Geometry check sheet. Reference: the model listing, model coordinates, mm. Face numbers are marked on the shaded views. A direction names the side the tool comes from. Coordinates: 2 decimals unless noted, no trailing zeros. Write each loop counter-clockwise with the first axis right and the second up, starting at its lowest first coordinate (ties: lowest second). Pieces come first, ordered by that corner, then holes. Notation, with made-up numbers: (69, 88) - (112, 88) arc R17 cw to (112, 101) - close; hole circle Ø11 at (9, 56). An arc over 180 degrees is marked (long way). Answer as a JSON object with one key per item and string values. Group by question number.
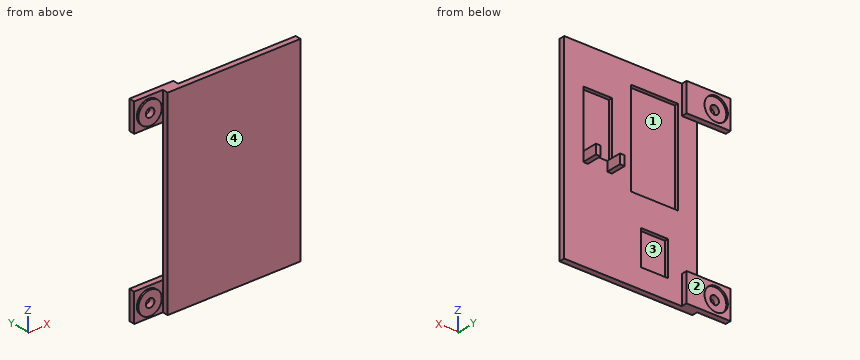
Autodesk Inventor part; units mm, degrees
ref_plane "YZ Plane" through (0, 0, 0) normal (1, 0, 0) x (0, 1, 0)
ref_plane "XZ Plane" through (0, 0, 0) normal (0, 1, 0) x (-1, 0, 0)
ref_plane "XY Plane" through (0, 0, 0) normal (0, 0, 1) x (1, 0, 0)
sketch "Sketch1" plane through (0, 0, 0) normal (0, 1, 0) x (-1, 0, 0)
  line L0 (7.25, 29.75) -> (-17.25, 29.75)
  line L1 (-17.25, 29.75) -> (-17.25, -19.75)
  line L2 (-17.25, -19.75) -> (7.25, -19.75)
  line L3 (7.25, -19.75) -> (7.25, 29.75)
  line L4 (7.25, 29.75) -> (-17.25, -19.75) construction
  line L5 (-17.25, 29.75) -> (7.25, -19.75) construction
  line L6 (-27.25, 20) -> (-42.25, 20)
  line L7 (-42.25, 20) -> (-42.25, -10)
  line L8 (-42.25, -10) -> (-27.25, -10)
  line L9 (-27.25, -10) -> (-27.25, 20)
  line L10 (-27.25, 20) -> (-42.25, -10) construction
  line L11 (-42.25, 20) -> (-27.25, -10) construction
  line L12 (2.1, -34.75) -> (-12.1, -34.75)
  line L13 (-12.1, -34.75) -> (-12.1, -52.95)
  line L14 (-12.1, -52.95) -> (2.1, -52.95)
  line L15 (2.1, -52.95) -> (2.1, -34.75)
  line L16 (2.1, -34.75) -> (-12.1, -52.95) construction
  line L17 (-12.1, -34.75) -> (2.1, -52.95) construction
  line L18 (17.25, 39.75) -> (17.25, -51.55)
  line L19 (17.25, 24.75) -> (17.25, 39.75)
  line L20 (17.25, -36.55) -> (17.25, -51.55)
  line L21 (17.25, 39.75) -> (-52.25, 39.75)
  line L22 (-52.25, 39.75) -> (-52.25, -63.35)
  line L23 (-52.25, -63.35) -> (17.25, -63.35)
  line L24 (17.25, -63.35) -> (17.25, 39.75)
  point P0 (-34.75, 5)
  point P1 (-5, -43.85)
  point P2 (17.25, 0)
  dimension "d0" = 24.5
  dimension "d1" = 49.5
  dimension "d2" = 15
  dimension "d3" = 30
  dimension "d4" = 10
  dimension "d7" = 14.2
  dimension "d8" = 18.2
  dimension "d9" = 15
  dimension "d17" = 10
  dimension "d19" = 103.1
  dimension "d21" = 10
  dimension "d22" = 10
extrude "Extrusion1" add sketch "Sketch1" along normal blind 3 contours L3 L2 L1 L0 | L9 L8 L7 L6 | L15 L14 L13 L12 | L18 L24 L23 L22 L21
sketch "Sketch2" plane through (0, 3, 0) normal (0, 1, 0) x (1, 0, 0)
  line L0 (-7.2398, -29.7311) -> (17.2602, -29.7311)
  line L1 (17.2602, -29.7311) -> (17.2602, 19.7689)
  line L2 (17.2602, 19.7689) -> (-7.2398, 19.7689)
  line L3 (-7.2398, 19.7689) -> (-7.2398, -29.7311)
  line L4 (-7.2398, -29.7311) -> (17.2602, 19.7689) construction
  line L5 (17.2602, -29.7311) -> (-7.2398, 19.7689) construction
  line L6 (27.2602, -19.9811) -> (42.2602, -19.9811)
  line L7 (42.2602, -19.9811) -> (42.2602, 10.0189)
  line L8 (42.2602, 10.0189) -> (27.2602, 10.0189)
  line L9 (27.2602, 10.0189) -> (27.2602, -19.9811)
  line L10 (27.2602, -19.9811) -> (42.2602, 10.0189) construction
  line L11 (42.2602, -19.9811) -> (27.2602, 10.0189) construction
  line L12 (-2.0898, 34.7689) -> (12.1102, 34.7689)
  line L13 (12.1102, 34.7689) -> (12.1102, 52.9689)
  line L14 (12.1102, 52.9689) -> (-2.0898, 52.9689)
  line L15 (-2.0898, 52.9689) -> (-2.0898, 34.7689)
  line L16 (-2.0898, 34.7689) -> (12.1102, 52.9689) construction
  line L17 (12.1102, 34.7689) -> (-2.0898, 52.9689) construction
  line L18 (-17.2398, -39.7311) -> (-17.2398, 51.5689)
  line L19 (-17.2398, -39.7311) -> (-32.2398, -39.7311)
  line L20 (-32.2398, -39.7311) -> (-32.2398, -24.7311)
  line L21 (-32.2398, -24.7311) -> (-17.2398, -24.7311)
  line L22 (-17.2398, -24.7311) -> (-17.2398, -39.7311)
  line L23 (-17.2398, 51.5689) -> (-32.2398, 51.5689)
  line L24 (-32.2398, 51.5689) -> (-32.2398, 36.5689)
  line L25 (-32.2398, 36.5689) -> (-17.2398, 36.5689)
  line L26 (-17.2398, 36.5689) -> (-17.2398, 51.5689)
  line L27 (-17.2398, -39.7311) -> (52.2602, -39.7311)
  line L28 (52.2602, -39.7311) -> (52.2602, 63.3689)
  line L29 (52.2602, 63.3689) -> (-17.2398, 63.3689)
  line L30 (-17.2398, 63.3689) -> (-17.2398, -39.7311)
  point P0 (0, 0)
  point P1 (34.7602, -4.9811)
  point P2 (5.0102, 43.8689)
  point P3 (-17.2398, 0.0189)
  dimension "d25" = 24.5
  dimension "d26" = 49.5
  dimension "d27" = 15
  dimension "d28" = 30
  dimension "d29" = 10
  dimension "d30" = 14.2
  dimension "d31" = 18.2
  dimension "d32" = 15
  dimension "d33" = 15
  dimension "d34" = 15
  dimension "d35" = 15
  dimension "d36" = 15
  dimension "d37" = 10
  dimension "d38" = 11.8
  dimension "d39" = 103.1
  dimension "d40" = 10
  dimension "d41" = 10
extrude "Extrusion2" cut sketch "Sketch2" against normal blind 2 contours L3 L2 L1 L0 | L9 L8 L7 L6 | L15 L14 L13 L12
sketch "Sketch3" plane through (0, 3, 0) normal (0, 1, 0) x (1, 0, 0)
  point P0 (0, 0)
sketch "Sketch4" plane through (0, 3, 0) normal (0, 1, 0) x (1, 0, 0)
  line L0 (29.7102, 15.7954) -> (39.8102, 15.7954)
  line L1 (39.8102, 15.7954) -> (39.8102, 4.2425)
  line L2 (39.8102, 4.2425) -> (29.7102, 4.2425)
  line L3 (29.7102, 4.2425) -> (29.7102, 15.7954)
  line L4 (27.2602, 10.0189) -> (42.2602, 10.0189)
  line L5 (29.7102, 15.7954) -> (39.8102, 4.2425) construction
  line L6 (39.8102, 15.7954) -> (29.7102, 4.2425) construction
  line L7 (27.2602, 10.0189) -> (29.7102, 10.0189)
  line L8 (29.7102, 10.0189) -> (29.7102, 15.0189)
  line L9 (29.7102, 15.0189) -> (27.2602, 15.0189)
  line L10 (27.2602, 15.0189) -> (27.2602, 10.0189)
  line L11 (42.2602, 10.0189) -> (39.8102, 10.0189)
  line L12 (39.8102, 10.0189) -> (39.8102, 15.0189)
  line L13 (39.8102, 15.0189) -> (42.2602, 15.0189)
  line L14 (42.2602, 15.0189) -> (42.2602, 10.0189)
  point P0 (0, 0)
  point P1 (34.7602, 10.0189)
  point P2 (39.8102, 10.0189)
  point P3 (29.7102, 10.0189)
  dimension "d44" = 10.1
  dimension "d45" = 5
  dimension "d46" = 5
extrude "Extrusion3" add sketch "Sketch4" along normal blind 8 contours L3 L4 L10 L9 | L13 L14 L4 L1
sketch "Sketch7" plane through (0, 3, 0) normal (0, 1, 0) x (1, 0, 0)
  line L0 (-17.25, -39.75) -> (-32.25, -39.75)
  line L1 (-32.25, -39.75) -> (-32.25, -24.75)
  line L2 (-32.25, -24.75) -> (-17.25, -24.75)
  line L3 (-17.25, -24.75) -> (-17.25, -39.75)
  line L4 (52.25, 63.35) -> (-17.25, 63.35)
  line L5 (-17.25, 63.35) -> (-32.25, 63.35)
  line L6 (-32.25, 63.35) -> (-32.25, 48.35)
  line L7 (-32.25, 48.35) -> (-17.25, 48.35)
  line L8 (-17.25, 48.35) -> (-17.25, 63.35)
  line L9 (-17.25, -39.75) -> (-9.25, -39.75)
  line L10 (-9.25, -39.75) -> (-9.25, -24.75)
  line L11 (-9.25, -24.75) -> (-17.25, -24.75)
  line L12 (-17.25, -24.75) -> (-17.25, -39.75)
  line L13 (-17.25, 48.35) -> (-9.25, 48.35)
  line L14 (-9.25, 48.35) -> (-9.25, 63.35)
  line L15 (-9.25, 63.35) -> (-17.25, 63.35)
  line L16 (-17.25, 63.35) -> (-17.25, 48.35)
  point P0 (0, 0)
  dimension "d52" = 15
  dimension "d53" = 15
  dimension "d54" = 15
  dimension "d55" = 15
  dimension "d56" = 8
extrude "Extrusion5" add sketch "Sketch7" along normal blind 3
sketch "Sketch8" plane through (0, 6, 0) normal (0, 1, 0) x (1, 0, 0)
  line L0 (-32.25, -24.75) -> (-32.25, -39.75)
  line L1 (-9.25, -24.75) -> (-32.25, -24.75)
  line L2 (-17.25, 63.35) -> (-17.25, -39.75)
  line L3 (-17.25, -24.75) -> (-32.25, -24.75)
  circle A0 centre (-24.75, -32.25) radius 2.25
  circle A1 centre (-24.75, 55.85) radius 2.25
  point P0 (0, 0)
  dimension "d59" = 4.5
  dimension "d60" = 4.5
extrude "Extrusion6" cut sketch "Sketch8" against normal blind 3
sketch "Sketch9" plane through (0, 6, 0) normal (0, 1, 0) x (1, 0, 0)
  circle A0 centre (-24.75, -32.25) radius 2.25
  circle A1 centre (-24.75, -32.25) radius 6.1
  circle A2 centre (-24.75, 55.85) radius 2.25
  circle A3 centre (-24.75, 55.85) radius 6.1
  point P0 (0, 0)
  dimension "d63" = 12.2
  dimension "d64" = 12.2
extrude "Extrusion7" cut sketch "Sketch9" against normal blind 1 contours A0 | A1 | A3
sketch "Sketch10" plane through (0, 3, 0) normal (0, -1, 0) x (1, 0, 0)
  circle A0 centre (-24.75, 32.25) radius 2.25
  circle A1 centre (-24.75, 32.25) radius 6.1
  circle A2 centre (-24.75, -55.85) radius 2.25
  circle A3 centre (-24.75, -55.85) radius 6.1
  point P0 (0, 0)
  dimension "d67" = 12.2
  dimension "d68" = 12.2
extrude "Extrusion8" add sketch "Sketch10" along normal blind 1
properties part number "chrager_adapter"
(1) Material ranges on L1, parallel to Z at x = -24.75, y = 5.3; L2, parallel to Z at x = -24.75, y = 3.55; L3, parallel to Z at x = 29, y = 2, recorded low to high. Write a range as [from, to].
(2) Gauge pin test, flat ends, axial feed: pin 1 (2 mm diameter, centred on y = 2, z = -1, fed in from -X); pin 2 (7.5 mm diameter, centred on x = 37, z = 5.5, fed in from +Y); pin 3 (3.5 mm diameter, centred on y = 5, z = -55.5, fed in from +X); pin 4 (6 mm diameter, centred on y = 7.5, z = -29.5, fed in from -X) (3 decimals). Record the tip position at first contact, or that the pin passes through.
(3) Set-up check for the marked faces 1 and 2: record each of +Z, -Z, +X, -X, +Y, -Y from which the full face is reachable in a straight line by a thin tool's end or side.
(4) Section check A-A (x = -24.75). Count the separate pieces of the cut face and the enclosed holes in it, and give its area (3 significant figures).
(5) Section check B-B (z = -55.85). Record the cut outline in (x, y), and give its area (3 significant figures).
(6) Section check C-C (y = 9.25). Record the cut outline in (x, z).
(7) Section check D-D (z = -38.5). Record the cut outline in (x, y), and give its area (3 significant figures).
(8) Draft check along Z on the marked faces 3 and 4. Enter one of: +Z half, -Z half, draft (parallel to the pull), parting line (faces both ways), or undercut.
Conclusion:
{
 "1": {"L1": "z = [-63.35, -61.95], [-49.75, -48.35], [24.75, 26.15], [38.35, 39.75]", "L2": "z = [-63.35, -58.1], [-53.6, -48.35], [24.75, 30], [34.5, 39.75]", "L3": "z = [-63.35, -10.02], [19.98, 39.75]"},
 "2": {"pin 1": "stops at x = -17.25", "pin 2": "stops at y = 1", "pin 3": "stops at x = -9.25", "pin 4": "passes through"},
 "3": {"face 1": "+Y", "face 2": "+Z, -Z, +X, -X, +Y"},
 "4": {"separate pieces": "4", "enclosed holes": "0", "area": "63.0 mm^2"},
 "5": {"outline": "(-32.25, 3) - (-30.85, 3) - (-30.85, 2) - (-27, 2) - (-27, 5) - (-30.85, 5) - (-30.85, 6) - (-32.25, 6) - close; (-22.5, 2) - (-18.65, 2) - (-18.65, 3) - (-17.25, 3) - (-17.25, 0) - (52.25, 0) - (52.25, 3) - (-9.25, 3) - (-9.25, 6) - (-18.65, 6) - (-18.65, 5) - (-22.5, 5) - close", "area": "264 mm^2"},
 "6": {"outline": "(27.26, -15.02) - (29.71, -15.02) - (29.71, -10.02) - (27.26, -10.02) - close; (39.81, -15.02) - (42.26, -15.02) - (42.26, -10.02) - (39.81, -10.02) - close"},
 "7": {"outline": "(-17.25, 0) - (52.25, 0) - (52.25, 3) - (12.11, 3) - (12.11, 1) - (-2.09, 1) - (-2.09, 3) - (-17.25, 3) - close", "area": "180 mm^2"},
 "8": {"face 3": "undercut", "face 4": "draft"}
}
